Can you work these out from the model? Positions are in its coordinate system, mm. A direction names the side the tool comes from. Coordinates: 2 decimals unless noted, no trailing zeros. Order: outer loops, then holes, each group sorted by start corner. A loop starts at its lowest first (then second) coordinate and runs counter-clockwise, first axis right, second up. Notation, with made-up numbers: (30, -26.5) -> (83, -26.5) arc R23 cw to (83, -3.5) -> close; hole circle Ø10 at (-27.75, 81). An arc over 180 degrees is marked (long way). Answer in a Markdown table with one row per item. Add a question column.
1. Imagine slicing it at B-B on z = -10.5. Write out the boundary of the cut face in (x, y) (1 decimal), plus the area to 3 significant figures.
2. Imagine slicing it at C-C on y = 15.75. Write out the boundary of the cut face in (x, z).
3. If I drill on line 1 along Y through (x, z) = (21, -6.5); line 2 along X through (y, z) = (17, -15.5), over which ranges is the centre line in solid material (lowest first)? Write a range as [from, to].
4. Imagine slicing it at A-A on z = -14.5. Write out the boundary of the cut face in (x, y) (1 decimal), plus the area to 3 significant figures.
5. Imagine slicing it at D-D on x = 15. Write out the boundary of the cut face in (y, z), plus the area to 3 significant figures.
6. We'd pull the mould along Y, two halves only. Please class faces 3 (the face through (24.6, 14.03, -10.92)), 4 (the face through (24, 6, 0)), 5 (the face through (11, -1.588, -10)): pulls with the +Y half, pulls with the -Y half, needs draft (parallel to the pull), parting line crosses it, or undercut.
7. On a 3-axis mill with a long thin cutter (end or side, diameter ignored), from which of +Z, -Z, +X, -X, +Y, -Y can I reach the whole of each face in a straight line? I mean faces 1 (the face through (11, 0, -10)), 2 (the face through (24.62, -0.85, -9.39)). Say none if no direction works.
8. Will these pins go through, and if not, where does the flat tip stop? pin 1 (3 mm diameter, centred on x = 21, z = -11, fed in from +Y); pin 2 (4 mm diameter, centred on x = 8.82, z = -9.66, fed in from -Y).
from build123d import *

# Parameters (mm, degrees)
SKETCH1_W                    = 25.4
SKETCH1_H                    = 19.05
BASE_FLANGE1_DEPTH           = 1.5875
EDGE_FLANGE1_STRIP_W         = 8.35
EDGE_FLANGE1_STRIP_H         = 1.5875
EDGE_FLANGE1_STRIP_CUT_DEPTH = 19.05
EDGE_FLANGE1_DEPTH           = 19.05
F_1_8_0_125_DIAMETER_HOLE1_D = 3.175
F_1_8_0_125_DIAMETER_HOLE2_D = 3.175


# Sheet-metal steps are written as plain solids
with BuildPart() as part:
    # Sketch1 → Base-Flange1 (new body)
    with BuildSketch(Plane(origin=(0, 0, 0), x_dir=(1, 0, 0), z_dir=(0, 1, 0))):
        with Locations((12.7, 9.525)):
            Rectangle(SKETCH1_W, SKETCH1_H)
    extrude(amount=-BASE_FLANGE1_DEPTH)

    # Edge-Flange1 strip (across the edge) → Edge-Flange1 strip cut (cut)
    with BuildSketch(Plane(origin=(25.4, 0, 0), x_dir=(-1, 0, 0), z_dir=(0, 0, -1))):
        with Locations((-1.5875, -0.79375)):
            Rectangle(EDGE_FLANGE1_STRIP_W, EDGE_FLANGE1_STRIP_H)
    extrude(amount=EDGE_FLANGE1_STRIP_CUT_DEPTH, mode=Mode.SUBTRACT)

    # Edge-Flange1 section (across the edge) → Edge-Flange1 (add)
    with BuildSketch(Plane(origin=(25.4, 0, 0), x_dir=(-1, 0, 0), z_dir=(0, 0, -1))):
        with BuildLine():
            Line((0, 1), (0, 23.8125))
            Line((0, 23.8125), (1.5875, 23.8125))
            Line((1.5875, 23.8125), (1.5875, 1))
            ThreePointArc((1.5875, 1), (1.880393219, 0.292893219), (2.5875, 0))
            Line((2.5875, 0), (2.5875, -1.5875))
            ThreePointArc((2.5875, -1.5875), (0.757861204, -0.829638796), (0, 1))
        make_face()
    extrude(amount=EDGE_FLANGE1_DEPTH)

    # 1/8 (0.125) Diameter Hole1 (through all)
    with Locations(Plane(origin=(25.4, 0, 0), x_dir=(0, 0, -1), z_dir=(1, 0, 0))):
        with Locations((9.658223344, 14.994606781)):
            Hole(F_1_8_0_125_DIAMETER_HOLE1_D / 2)

    # 1/8 (0.125) Diameter Hole2 (through all)
    with Locations(Plane(origin=(0, -1.5875, 0), x_dir=(-1, 0, 0), z_dir=(0, -1, 0))):
        with Locations((-8.817893219, 9.658223344)):
            Hole(F_1_8_0_125_DIAMETER_HOLE2_D / 2)


solid = part.part
Answers follow:
| question | item | result |
|---|---|---|
| 1 | outline | (0, -1.6) -> (7.5, -1.6) -> (7.5, 0) -> (0, 0) -> close; (10.2, -1.6) -> (22.8, -1.6) arc R2.6 ccw to (25.4, 1) -> (25.4, 13.6) -> (23.8, 13.6) -> (23.8, 1) arc R1 cw to (22.8, 0) -> (10.2, 0) -> close; (23.8, 16.3) -> (25.4, 16.3) -> (25.4, 23.8) -> (23.8, 23.8) -> close |
| 1 | area | 68.4 mm² |
| 2 | outline | (23.81, -19.05) -> (25.4, -19.05) -> (25.4, -11.05) -> (23.81, -11.05) -> close; (23.81, -8.26) -> (25.4, -8.26) -> (25.4, 0) -> (23.81, 0) -> close |
| 3 | line 1 | y = [-1.59, 0] |
| 3 | line 2 | x = [23.81, 25.4] |
| 4 | outline | (0, -1.6) -> (22.8, -1.6) arc R2.6 ccw to (25.4, 1) -> (25.4, 23.8) -> (23.8, 23.8) -> (23.8, 1) arc R1 cw to (22.8, 0) -> (0, 0) -> close |
| 4 | area | 76.9 mm² |
| 5 | outline | (-1.59, -19.05) -> (0, -19.05) -> (0, 0) -> (-1.59, 0) -> close |
| 5 | area | 30.2 mm² |
| 6 | face 3 | undercut |
| 6 | face 4 | needs draft |
| 6 | face 5 | pulls with the -Y half |
| 7 | face 1 | +Z, -Z, -X, +Y |
| 7 | face 2 | +Z, -Z, +X, -Y |
| 8 | pin 1 | stops at y = 0 |
| 8 | pin 2 | stops at y = -1.59 |
